The model under review builds one solid part; all positions refer to its coordinate system, in mm. Face numbers are marked on the shaded views. A direction names the side the tool comes from. Round coordinates to 2 decimals unless told otherwise and drop trailing zeros. Order: outer loops, then holes, each group sorted by start corner. A loop starts at its lowest first (then second) coordinate and runs counter-clockwise, first axis right, second up. Notation, with made-up numbers: M 17,19.5 L 43,19.5 A21 ccw 43,27.5 Z; hole C -10.75,-37 d10. An arc over 180 degrees is marked long. Answer as a JSON object with one key per item and string values. Group by question number.
1) Consider section B-B, the plane z = 4.25. Write out the cut boundary in (x, y), then the cut area to 3 significant figures.
2) For the marked faces 1, 2 and 3, list the 3-axis set-ups (+Z, -Z, +X, -X, +Y, -Y) from which the entire face can be reached by the end or side of a thin tool; tool diameter is ignored.
3) To check wall thickness, follow line 1 (Y direction, x = -4, z = 8.25); line 2 (X direction, y = 12.75, z = 6.75); line 3 (Y direction, x = -5.5, z = 6). State the ranges of each line that lie inside material, in increasing order.
4) Consider section C-C, the plane y = 9.25. Write out the cut boundary in (x, z).
5) Insertion check: pin 1 Ø1.8 at (x, y) = (-4.5, 14) entering from +Z; pin 2 Ø1.5 at (y, z) = (10, 7) entering from +X; pin 3 Ø0.6 at (y, z) = (10.5, 7.5) entering from -X. Each pin has a flat end and moves straight along its axis. Give the tip position at first contact, or say it passes through.
6) Consider section A-A, the plane z = 6.25. Write out the cut boundary in (x, y).
7) Consider section D-D, the plane x = -1.5. Write out the cut boundary in (y, z), then the cut area to 3 significant figures.
```python
from build123d import *

# Parameters (mm, degrees)
F0_R     = 3
F1_DEPTH = 2.8
F2_DEPTH = 4
F3_ANGLE = 180


with BuildPart() as f1:
    # F0 (on Top) → F1 (new body)
    with BuildSketch(Plane.XY):
        with BuildLine():
            Line((0, 12.7), (0, 0))
            Line((0, 0), (-0.2, -0.4))
            Line((-0.2, -0.4), (8, -0.4))
            Line((8, -0.4), (7.8, 0))
            Line((7.8, 0), (7.8, 12.7))
            ThreePointArc((7.8, 12.7), (6.6577164466, 15.4577164466), (3.9, 16.6))
            ThreePointArc((3.9, 16.6), (1.1422835534, 15.4577164466), (0, 12.7))
        make_face()
        with Locations((3.9, 12.7)):
            Circle(F0_R, mode=Mode.SUBTRACT)
        with Locations((3.9, 12.7)):
            Circle(F0_R)
        with BuildLine():
            ThreePointArc((3.9, 10.1), (3.6488251879, 10.1121608988), (3.4, 10.1485298356))
            ThreePointArc((3.4, 10.1485298356), (2.2477288358, 14.70748599), (6.5, 12.7))
            ThreePointArc((6.5, 12.7), (5.7384776311, 10.8615223689), (3.9, 10.1))
        make_face(mode=Mode.SUBTRACT)
        with BuildLine():
            ThreePointArc((3.9, 10.6), (5.3849242405, 11.2150757595), (6, 12.7))
            ThreePointArc((6, 12.7), (2.6038518603, 14.3522711642), (3.4, 10.6603921946))
            ThreePointArc((3.4, 10.6603921946), (3.6481829944, 10.6151527165), (3.9, 10.6))
        make_face()
        with BuildLine():
            ThreePointArc((3.4, 10.6603921946), (2.6038518603, 14.3522711642), (6, 12.7))
            ThreePointArc((6, 12.7), (5.3849242405, 11.2150757595), (3.9, 10.6))
            Line((3.9, 10.6), (3.9, 10.1))
            ThreePointArc((3.9, 10.1), (5.7384776311, 10.8615223689), (6.5, 12.7))
            ThreePointArc((6.5, 12.7), (2.2477288358, 14.70748599), (3.4, 10.1485298356))
            Line((3.4, 10.1485298356), (3.4, 10.6603921946))
        make_face()
        with BuildLine():
            ThreePointArc((3.9, 10.6), (3.6481829944, 10.6151527165), (3.4, 10.6603921946))
            Line((3.4, 10.6603921946), (3.4, 10.1485298356))
            ThreePointArc((3.4, 10.1485298356), (3.6488251879, 10.1121608988), (3.9, 10.1))
            Line((3.9, 10.1), (3.9, 10.6))
        make_face()
    extrude(amount=F1_DEPTH)

    # F0 (on Top) → F2 (join)
    with BuildSketch(Plane.XY):
        with BuildLine():
            Line((0, 12.7), (0, 0))
            Line((0, 0), (-0.2, -0.4))
            Line((-0.2, -0.4), (8, -0.4))
            Line((8, -0.4), (7.8, 0))
            Line((7.8, 0), (7.8, 12.7))
            ThreePointArc((7.8, 12.7), (6.6577164466, 15.4577164466), (3.9, 16.6))
            ThreePointArc((3.9, 16.6), (1.1422835534, 15.4577164466), (0, 12.7))
        make_face()
        with Locations((3.9, 12.7)):
            Circle(F0_R, mode=Mode.SUBTRACT)
        with BuildLine():
            ThreePointArc((3.4, 10.6603921946), (2.6038518603, 14.3522711642), (6, 12.7))
            ThreePointArc((6, 12.7), (5.3849242405, 11.2150757595), (3.9, 10.6))
            Line((3.9, 10.6), (3.9, 10.1))
            ThreePointArc((3.9, 10.1), (5.7384776311, 10.8615223689), (6.5, 12.7))
            ThreePointArc((6.5, 12.7), (2.2477288358, 14.70748599), (3.4, 10.1485298356))
            Line((3.4, 10.1485298356), (3.4, 10.6603921946))
        make_face()
    extrude(amount=-F2_DEPTH)


with BuildPart() as f1_1:
    # F3: moved
    add(f1.part.rotate(Axis((0, 6.35, 2.8), (0, 1, 0)), F3_ANGLE))


solid = f1_1.part
```
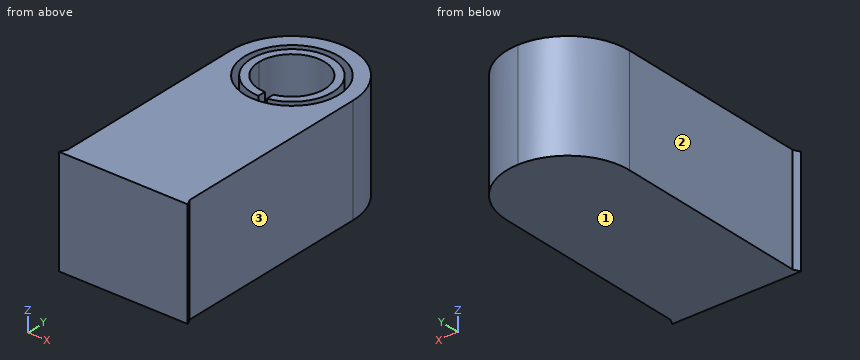
Results list:
{
 "1": {"outline": "M -8,-0.4 L 0.2,-0.4 L 0,0 L 0,12.7 A3.9 ccw -7.8,12.7 L -7.8,0 Z", "area": "126 mm^2"},
 "2": {"face 1": "-Z, +X, -X, +Y, -Y", "face 2": "+Z, -Z, -X, +Y", "face 3": "+Z, -Z, +X, +Y"},
 "3": {"line 1": "-0.4 to 9.7, 10.1 to 10.6, 14.8 to 15.3, 15.7 to 16.6", "line 2": "-7.8 to -6.9, -6.5 to -6, -1.8 to -1.3, -0.9 to 0", "line 3": "-0.4 to 10.16, 10.65 to 11.34, 14.06 to 14.75, 15.24 to 16.26"},
 "4": {"outline": "M -7.8,2.8 L 0,2.8 L 0,9.6 L -7.8,9.6 Z"},
 "5": {"pin 1": "z = 9.6", "pin 2": "x = 0", "pin 3": "x = -7.8"},
 "6": {"outline": "M -8,-0.4 L 0.2,-0.4 L 0,0 L 0,12.7 A3.9 ccw -7.8,12.7 L -7.8,0 Z; M -3.9,10.1 L -3.9,10.6 A2.1 cw long -3.4,10.66 L -3.4,10.15 A2.6 ccw long Z; hole C -3.9,12.7 d6"},
 "7": {"outline": "M -0.4,2.8 L 15.77,2.8 L 15.77,9.6 L 14.5,9.6 L 14.5,5.6 L 13.7,5.6 L 13.7,9.6 L 11.7,9.6 L 11.7,5.6 L 10.9,5.6 L 10.9,9.6 L -0.4,9.6 Z", "area": "104 mm^2"}
}
